Input: part model. Units: mm. Frame: model coordinates. Give positions to 0.01 mm unless a question says otherwise; leave off trailing zeros. Write each loop counter-clockwise with the first axis right and the second up, starting at its lowest first coordinate (ties: lowest second). Pieces come first, ordered by that corner, then holes. Notation, with made-up numbers: (49.25, 50) - (104.25, 50) arc R15 ccw to (104.25, 64) - close; hole circle Ø2 at (81.25, 82). An arc over 180 degrees is marked (long way). Use a Markdown table: item, result. Add a question column.
1. Section query A-A, the plane z = 0. Return loops of the section in (x, y).
2. Section query B-B, the plane x = 81.28. Return loops of the section in (y, z), plus the area to 3 significant figures.
3. Mould query, pull axis X, two halves, no side actions, for faces 1 (the flat face through (-101.6, 13, 0)), 2 (the cylindrical face through (84.4, 12.9, 1.3)), 3 (the flat face through (-1, 25.4, -5)). Classes: released by +X, released by -X, zero draft, split by the parting line, or undercut.
4. Material intervals for probe 1 along X at (y, z) = (11, 0); probe 2 along Z at (x, y) = (0, 18.75); probe 3 along X at (y, z) = (21.75, 3), sorted ascending.
5. Pin query (flat end, axial travel): pin 1 (4 mm diameter, centred on x = 81.28, z = 0, fed in from +Y). Return the tip coordinate at first contact, or that it passes through.
```python
from build123d import *

# Parameters (mm, degrees)
SKETCH1_W           = 203.2
SKETCH1_H           = 38.1
BOSS_EXTRUDE1_DEPTH = 25.4
SKETCH2_R           = 3.3782
CUT_EXTRUDE1_DEPTH  = 26.4


with BuildPart() as part:
    # Sketch1 → Boss-Extrude1 (new body)
    with BuildSketch(Plane(origin=(0, 0, 0), x_dir=(1, 0, 0), z_dir=(0, 1, 0))):
        Rectangle(SKETCH1_W, SKETCH1_H)
    extrude(amount=BOSS_EXTRUDE1_DEPTH)

    # Sketch2 → Cut-Extrude1 (cut, through all)
    with BuildSketch(Plane(origin=(0, 25.4, 0), x_dir=(1, 0, 0), z_dir=(0, 1, 0))):
        Circle(SKETCH2_R)
        with Locations((-81.28, 0)):
            Circle(SKETCH2_R)
        with Locations((81.28, 0)):
            Circle(SKETCH2_R)
    extrude(amount=-CUT_EXTRUDE1_DEPTH, mode=Mode.SUBTRACT)


solid = part.part
```
Result sheet:
| question | item | result |
|---|---|---|
| 1 | outline | (-101.6, 0) - (-84.66, 0) - (-84.66, 25.4) - (-101.6, 25.4) - close; (-77.9, 0) - (-3.38, 0) - (-3.38, 25.4) - (-77.9, 25.4) - close; (3.38, 0) - (77.9, 0) - (77.9, 25.4) - (3.38, 25.4) - close; (84.66, 0) - (101.6, 0) - (101.6, 25.4) - (84.66, 25.4) - close |
| 2 | outline | (0, -19.05) - (25.4, -19.05) - (25.4, -3.38) - (0, -3.38) - close; (0, 3.38) - (25.4, 3.38) - (25.4, 19.05) - (0, 19.05) - close |
| 2 | area | 796 mm² |
| 3 | face 1 | released by -X |
| 3 | face 2 | undercut |
| 3 | face 3 | zero draft |
| 4 | probe 1 | x = -101.6 to -84.66, -77.9 to -3.38, 3.38 to 77.9, 84.66 to 101.6 |
| 4 | probe 2 | z = -19.05 to -3.38, 3.38 to 19.05 |
| 4 | probe 3 | x = -101.6 to -82.83, -79.73 to -1.55, 1.55 to 79.73, 82.83 to 101.6 |
| 5 | pin 1 | passes through |
